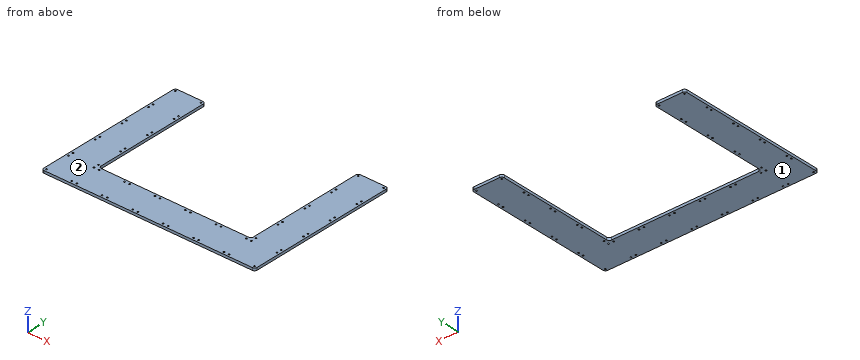
Autodesk Inventor part; units mm, degrees
ref_plane "YZ Plane" through (0, 0, 0) normal (1, 0, 0) x (0, 1, 0)
ref_plane "XZ Plane" through (0, 0, 0) normal (0, 1, 0) x (-1, 0, 0)
ref_plane "XY Plane" through (0, 0, 0) normal (0, 0, 1) x (1, 0, 0)
sketch "Sketch1" plane through (0, 0, 0) normal (0, 0, 1) x (1, 0, 0)
  line L0 (0, 0) -> (420, 0)
  line L1 (420, 0) -> (420, 300)
  line L2 (420, 300) -> (360, 300)
  line L3 (360, 300) -> (360, 60)
  line L4 (360, 60) -> (60, 60)
  line L5 (60, 60) -> (60, 300)
  line L6 (60, 300) -> (0, 300)
  line L7 (0, 300) -> (0, 0)
  line L8 (0, 300) -> (0, 240) construction
  line L9 (0, 240) -> (0, 180) construction
  line L10 (0, 180) -> (0, 120) construction
  line L11 (0, 120) -> (0, 60) construction
  line L12 (420, 300) -> (420, 240) construction
  line L13 (420, 240) -> (420, 180) construction
  line L14 (420, 180) -> (420, 120) construction
  line L15 (420, 120) -> (420, 60) construction
  line L16 (60, 60) -> (120, 60) construction
  line L17 (120, 60) -> (180, 60) construction
  line L18 (180, 60) -> (240, 60) construction
  line L19 (240, 60) -> (300, 60) construction
  line L20 (300, 60) -> (360, 60) construction
  line L21 (0, 240) -> (60, 300) construction
  line L22 (0, 240) -> (60, 240) construction
  line L23 (0, 180) -> (60, 180) construction
  line L24 (0, 120) -> (60, 120) construction
  line L25 (0, 60) -> (60, 60) construction
  line L26 (60, 60) -> (60, 0) construction
  line L27 (0, 180) -> (60, 240) construction
  line L28 (0, 120) -> (60, 180) construction
  line L29 (0, 60) -> (60, 120) construction
  line L30 (0, 0) -> (60, 60) construction
  line L31 (120, 60) -> (120, 0) construction
  line L32 (180, 60) -> (180, 0) construction
  line L33 (240, 60) -> (240, 0) construction
  line L34 (300, 60) -> (300, 0) construction
  line L35 (360, 60) -> (360, 0) construction
  line L36 (360, 60) -> (420, 60) construction
  line L37 (360, 120) -> (420, 120) construction
  line L38 (420, 180) -> (360, 180) construction
  line L39 (420, 240) -> (360, 240) construction
  line L40 (60, 0) -> (120, 60) construction
  line L41 (120, 0) -> (180, 60) construction
  line L42 (180, 0) -> (240, 60) construction
  line L43 (240, 0) -> (300, 60) construction
  line L44 (300, 0) -> (360, 60) construction
  line L45 (360, 0) -> (420, 60) construction
  line L46 (360, 60) -> (420, 120) construction
  line L47 (360, 120) -> (420, 180) construction
  line L48 (360, 180) -> (420, 240) construction
  line L49 (360, 240) -> (420, 300) construction
  line L50 (5, 245) -> (55, 245) construction
  line L51 (55, 245) -> (55, 295) construction
  line L52 (55, 295) -> (5, 295) construction
  line L53 (5, 295) -> (5, 245) construction
  line L54 (5, 245) -> (55, 295) construction
  line L55 (55, 245) -> (5, 295) construction
  line L56 (5, 185) -> (55, 185) construction
  line L57 (55, 185) -> (55, 235) construction
  line L58 (55, 235) -> (5, 235) construction
  line L59 (5, 235) -> (5, 185) construction
  line L60 (5, 185) -> (55, 235) construction
  line L61 (55, 185) -> (5, 235) construction
  line L62 (5, 125) -> (55, 125) construction
  line L63 (55, 125) -> (55, 175) construction
  line L64 (55, 175) -> (5, 175) construction
  line L65 (5, 175) -> (5, 125) construction
  line L66 (5, 125) -> (55, 175) construction
  line L67 (55, 125) -> (5, 175) construction
  line L68 (5, 65) -> (55, 65) construction
  line L69 (55, 65) -> (55, 115) construction
  line L70 (55, 115) -> (5, 115) construction
  line L71 (5, 115) -> (5, 65) construction
  line L72 (5, 65) -> (55, 115) construction
  line L73 (55, 65) -> (5, 115) construction
  line L74 (5, 5) -> (55, 5) construction
  line L75 (55, 5) -> (55, 55) construction
  line L76 (55, 55) -> (5, 55) construction
  line L77 (5, 55) -> (5, 5) construction
  line L78 (5, 5) -> (55, 55) construction
  line L79 (55, 5) -> (5, 55) construction
  line L80 (65, 5) -> (115, 5) construction
  line L81 (115, 5) -> (115, 55) construction
  line L82 (115, 55) -> (65, 55) construction
  line L83 (65, 55) -> (65, 5) construction
  line L84 (65, 5) -> (115, 55) construction
  line L85 (115, 5) -> (65, 55) construction
  line L86 (125, 5) -> (175, 5) construction
  line L87 (175, 5) -> (175, 55) construction
  line L88 (175, 55) -> (125, 55) construction
  line L89 (125, 55) -> (125, 5) construction
  line L90 (125, 5) -> (175, 55) construction
  line L91 (175, 5) -> (125, 55) construction
  line L92 (185, 5) -> (235, 5) construction
  line L93 (235, 5) -> (235, 55) construction
  line L94 (235, 55) -> (185, 55) construction
  line L95 (185, 55) -> (185, 5) construction
  line L96 (185, 5) -> (235, 55) construction
  line L97 (235, 5) -> (185, 55) construction
  line L98 (245, 5) -> (295, 5) construction
  line L99 (295, 5) -> (295, 55) construction
  line L100 (295, 55) -> (245, 55) construction
  line L101 (245, 55) -> (245, 5) construction
  line L102 (245, 5) -> (295, 55) construction
  line L103 (295, 5) -> (245, 55) construction
  line L104 (305, 5) -> (355, 5) construction
  line L105 (355, 5) -> (355, 55) construction
  line L106 (355, 55) -> (305, 55) construction
  line L107 (305, 55) -> (305, 5) construction
  line L108 (305, 5) -> (355, 55) construction
  line L109 (355, 5) -> (305, 55) construction
  line L110 (365, 5) -> (415, 5) construction
  line L111 (415, 5) -> (415, 55) construction
  line L112 (415, 55) -> (365, 55) construction
  line L113 (365, 55) -> (365, 5) construction
  line L114 (365, 5) -> (415, 55) construction
  line L115 (415, 5) -> (365, 55) construction
  line L116 (365, 65) -> (415, 65) construction
  line L117 (415, 65) -> (415, 115) construction
  line L118 (415, 115) -> (365, 115) construction
  line L119 (365, 115) -> (365, 65) construction
  line L120 (365, 65) -> (415, 115) construction
  line L121 (415, 65) -> (365, 115) construction
  line L122 (365, 125) -> (415, 125) construction
  line L123 (415, 125) -> (415, 175) construction
  line L124 (415, 175) -> (365, 175) construction
  line L125 (365, 175) -> (365, 125) construction
  line L126 (365, 125) -> (415, 175) construction
  line L127 (415, 125) -> (365, 175) construction
  line L128 (365, 185) -> (415, 185) construction
  line L129 (415, 185) -> (415, 235) construction
  line L130 (415, 235) -> (365, 235) construction
  line L131 (365, 235) -> (365, 185) construction
  line L132 (365, 185) -> (415, 235) construction
  line L133 (415, 185) -> (365, 235) construction
  line L134 (365, 245) -> (415, 245) construction
  line L135 (415, 245) -> (415, 295) construction
  line L136 (415, 295) -> (365, 295) construction
  line L137 (365, 295) -> (365, 245) construction
  line L138 (365, 245) -> (415, 295) construction
  line L139 (415, 245) -> (365, 295) construction
  circle A0 centre (5, 295) radius 1.5
  circle A1 centre (55, 295) radius 1.5
  circle A2 centre (55, 245) radius 1.5
  circle A3 centre (5, 245) radius 1.5
  circle A4 centre (5, 5) radius 1.5
  circle A5 centre (55, 5) radius 1.5
  circle A6 centre (5, 55) radius 1.5
  circle A7 centre (55, 55) radius 1.5
  circle A8 centre (235, 55) radius 1.5
  circle A9 centre (185, 55) radius 1.5
  circle A10 centre (185, 5) radius 1.5
  circle A11 centre (235, 5) radius 1.5
  circle A12 centre (365, 55) radius 1.5
  circle A13 centre (415, 55) radius 1.5
  circle A14 centre (415, 5) radius 1.5
  circle A15 centre (365, 5) radius 1.5
  circle A16 centre (365, 295) radius 1.5
  circle A17 centre (415, 295) radius 1.5
  circle A18 centre (365, 245) radius 1.5
  circle A19 centre (415, 245) radius 1.5
  circle A20 centre (365, 235) radius 1.5
  circle A21 centre (415, 235) radius 1.5
  circle A22 centre (365, 185) radius 1.5
  circle A23 centre (415, 185) radius 1.5
  circle A24 centre (365, 175) radius 1.5
  circle A25 centre (415, 175) radius 1.5
  circle A26 centre (365, 125) radius 1.5
  circle A27 centre (415, 125) radius 1.5
  circle A28 centre (365, 115) radius 1.5
  circle A29 centre (415, 115) radius 1.5
  circle A30 centre (365, 65) radius 1.5
  circle A31 centre (415, 65) radius 1.5
  circle A32 centre (305, 55) radius 1.5
  circle A33 centre (355, 55) radius 1.5
  circle A34 centre (305, 5) radius 1.5
  circle A35 centre (355, 5) radius 1.5
  circle A36 centre (295, 55) radius 1.5
  circle A37 centre (245, 55) radius 1.5
  circle A38 centre (245, 5) radius 1.5
  circle A39 centre (295, 5) radius 1.5
  circle A40 centre (175, 55) radius 1.5
  circle A41 centre (125, 55) radius 1.5
  circle A42 centre (125, 5) radius 1.5
  circle A43 centre (175, 5) radius 1.5
  circle A44 centre (115, 55) radius 1.5
  circle A45 centre (65, 55) radius 1.5
  circle A46 centre (65, 5) radius 1.5
  circle A47 centre (115, 5) radius 1.5
  circle A48 centre (5, 65) radius 1.5
  circle A49 centre (55, 65) radius 1.5
  circle A50 centre (55, 115) radius 1.5
  circle A51 centre (5, 115) radius 1.5
  circle A52 centre (5, 125) radius 1.5
  circle A53 centre (55, 125) radius 1.5
  circle A54 centre (5, 175) radius 1.5
  circle A55 centre (55, 175) radius 1.5
  circle A56 centre (5, 185) radius 1.5
  circle A57 centre (55, 185) radius 1.5
  circle A58 centre (5, 235) radius 1.5
  circle A59 centre (55, 235) radius 1.5
  point P0 (30, 270)
  point P1 (30, 210)
  point P2 (30, 150)
  point P3 (30, 90)
  point P4 (30, 30)
  point P5 (90, 30)
  point P6 (150, 30)
  point P7 (210, 30)
  point P8 (270, 30)
  point P9 (330, 30)
  point P10 (390, 30)
  point P11 (390, 90)
  point P12 (390, 150)
  point P13 (390, 210)
  point P14 (390, 270)
  dimension "d0" = 420
  dimension "d1" = 300
  dimension "d2" = 60
  dimension "d3" = 240
  dimension "d4" = 300
  dimension "d5" = 240
  dimension "d6" = 60
  dimension "d7" = 60
  dimension "d8" = 60
  dimension "d9" = 60
  dimension "d10" = 60
  dimension "d11" = 60
  dimension "d12" = 60
  dimension "d13" = 60
  dimension "d14" = 60
  dimension "d15" = 60
  dimension "d16" = 60
  dimension "d17" = 60
  dimension "d20" = 50
  dimension "d21" = 50
  dimension "d22" = 50
  dimension "d23" = 50
  dimension "d24" = 50
  dimension "d25" = 50
  dimension "d26" = 50
  dimension "d27" = 50
  dimension "d28" = 50
  dimension "d29" = 50
  dimension "d30" = 50
  dimension "d31" = 50
  dimension "d32" = 50
  dimension "d33" = 50
  dimension "d34" = 50
  dimension "d35" = 50
  dimension "d36" = 50
  dimension "d37" = 50
  dimension "d38" = 50
  dimension "d39" = 50
  dimension "d40" = 50
  dimension "d41" = 50
  dimension "d42" = 50
  dimension "d43" = 50
  dimension "d44" = 50
  dimension "d45" = 50
  dimension "d46" = 50
  dimension "d47" = 50
  dimension "d48" = 50
  dimension "d49" = 50
  dimension "d50" = 3
  dimension "d51" = 3
  dimension "d52" = 3
  dimension "d53" = 3
  dimension "d54" = 3
  dimension "d55" = 3
  dimension "d56" = 3
  dimension "d57" = 3
  dimension "d58" = 3
  dimension "d59" = 3
  dimension "d60" = 3
  dimension "d61" = 3
  dimension "d62" = 3
  dimension "d63" = 3
  dimension "d64" = 3
  dimension "d65" = 3
extrude "Frame" add sketch "Sketch1" along normal blind 5
fillet "Fillet1" radius 5 8 edges at (60, 60, 2.5) (360, 60, 2.5) (420, 0, 2.5) (360, 300, 2.5) (420, 300, 2.5) (0, 0, 2.5) (0, 300, 2.5) (60, 300, 2.5)
properties part number "OuterFrame"
Build history of the part. All positions in model axes, mm. Face numbers are marked on the shaded views. Give positions to 0.01 mm unless a question says otherwise; leave off trailing zeros. Order: outer loops, then holes, each group sorted by start corner. A loop starts at its lowest first (then second) coordinate and runs counter-clockwise, first axis right, second up. Notation, with made-up numbers: M 17.5,52.25 L 30.5,52.25 A19 cw 30.5,75.25 Z; hole C 82,84 d4. An arc over 180 degrees is marked long. Use one line per item in the form item = value.
1) Saw through at A-A (y = 151.5). Give the cut face in (x, z), plus the area to 3 significant figures.
Calculated:
outline = M 0,0 L 60,0 L 60,5 L 0,5 Z; M 360,0 L 420,0 L 420,5 L 360,5 Z
area = 600 mm2
2) Probe probe 1 along X at (y, z) = (175, 1.95); probe 2 along X at (y, z) = (175.5, 3.65); probe 3 along X at (y, z) = (228, 0.35). List the from-to ranges inside material, lowest first.
Calculated:
probe_1 = 0 to 3.5, 6.5 to 53.5, 56.5 to 60, 360 to 363.5, 366.5 to 413.5, 416.5 to 420
probe_2 = 0 to 3.59, 6.41 to 53.59, 56.41 to 60, 360 to 363.59, 366.41 to 413.59, 416.41 to 420
probe_3 = 0 to 60, 360 to 420
3) Drop flat-ended pins along their axis: pin 1 (4 mm diameter, centred on x = 5, y = 55, fed in from -Z); pin 2 (2.5 mm diameter, centred on x = 235, y = 55, fed in from -Z). Give the stop position or say it passes through.
Calculated:
pin_1 = 0
pin_2 = through
4) Two-plate mould, pull along Z, no slides. Class the marked faces 1 and 2: released by +Z, released by -Z, zero draft, split by the parting line, or undercut.
Calculated:
face_1 = released by -Z
face_2 = released by +Z
5) Saw through at C-C (x = 213.5). Give the cut face in (y, z), plus the area to 3 significant figures.
Calculated:
outline = M 0,0 L 60,0 L 60,5 L 0,5 Z
area = 300 mm2
6) Saw through at B-B (z = 2.65). State how many separate pieces and enclosed holes the cut face has, plus the area to 3 significant figures.
Calculated:
separate_pieces = 1
enclosed_holes = 60
area = 53,600 mm2
